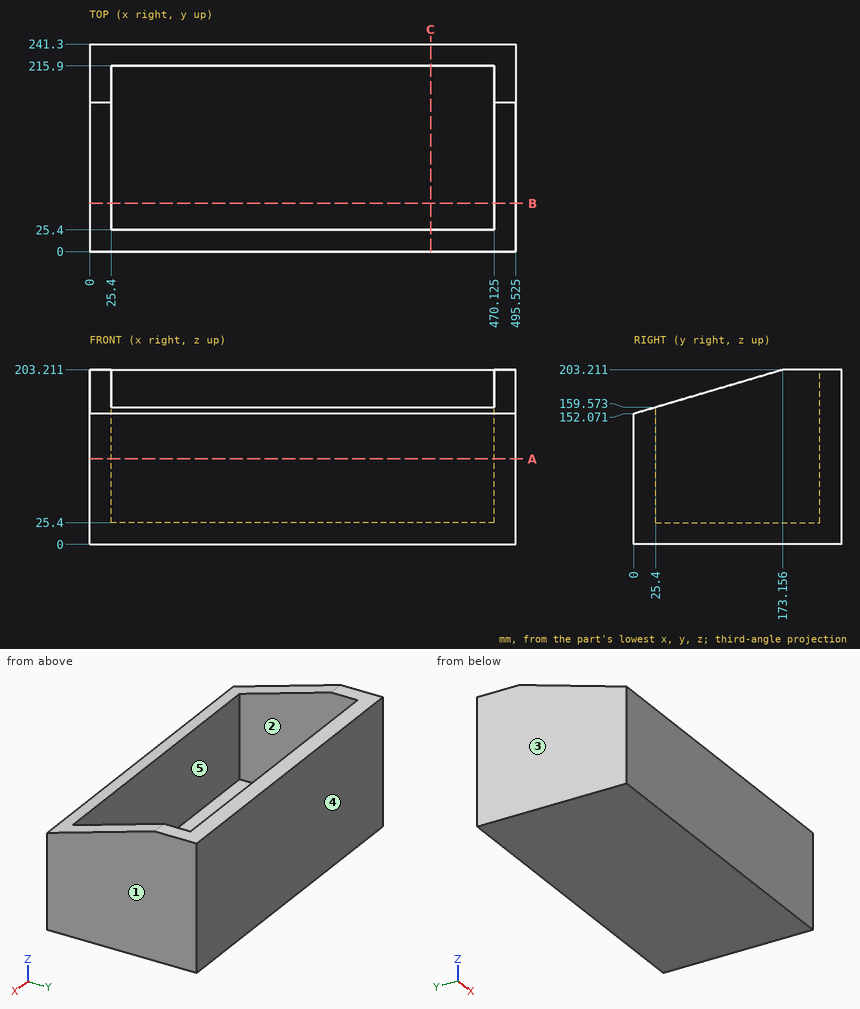
Design review of the part shown in the three views and the two pictorial views. Dimensions are in mm from the part's minimum x, y and z. A direction names the side the tool comes from. Give positions to 0.01 mm unless a question says otherwise; leave off trailing zeros. Loops run counter-clockwise (first coordinate to the right, second up) from the corner with the lowest first, then second, coordinate; pieces in that order, holes last. Notation, with made-up numbers: (53.5, -9.75) -> (107.5, -9.75) arc R19 ccw to (107.5, 8.25) -> close; hole circle Ø7 at (-2, 8.25). An arc over 180 degrees is marked (long way). Write each question's results on one line, items separated by ' | '.
1) Take a section at A-A, the plane z = 99.5. Give the boundary of the cut face in (x, y) (1 decimal), plus the area to 4 significant figures.
Conclusion:
outline: (0, 0) -> (495.5, 0) -> (495.5, 241.3) -> (0, 241.3) -> close; hole (25.4, 25.4) -> (470.1, 25.4) -> (470.1, 215.9) -> (25.4, 215.9) -> close | area: 34,850 mm^2
2) Take a section at B-B, the plane y = 56. Give the boundary of the cut face in (x, z) (1 decimal), plus the area to 3 significant figures.
Conclusion:
outline: (0, 0) -> (495.5, 0) -> (495.5, 168.6) -> (470.1, 168.6) -> (470.1, 25.4) -> (25.4, 25.4) -> (25.4, 168.6) -> (0, 168.6) -> close | area: 19,900 mm^2
3) Take a section at C-C, the plane x = 396.5. Give the boundary of the cut face in (y, z).
Conclusion:
outline: (0, 0) -> (241.3, 0) -> (241.3, 203.21) -> (215.9, 203.21) -> (215.9, 25.4) -> (25.4, 25.4) -> (25.4, 159.57) -> (0, 152.07) -> close
4) Insertion check: pin 1 Ø1.5 at (x, y) = (266.5, 96.5) entering from +Z. The pin has a flat end and moves straight along its axis. Give the tip position at first contact, or say it passes through.
Conclusion:
pin 1: stops at z = 25.4
5) For line 1 along X through (y, z) = (159, 112.5) (1 decimal); line 2 along Y through (x, z) = (83.5, 143.5); line 3 along Z through (x, y) = (44, 55.5), list the stretches that pass through material, from the lowest coordinate up. Write a range as from..to.
Conclusion:
line 1: x = 0..25.4, 470.1..495.5 | line 2: y = 0..25.4, 215.9..241.3 | line 3: z = 0..25.4
6) Draft analysis for pull direction X (two halves, no side actions). For the marked faces 1, 2 and 3, state which applies: pulls with the +X half, pulls with the -X half, needs draft (parallel to the pull), parting line crosses it, or undercut.
Conclusion:
face 1: pulls with the +X half | face 2: undercut | face 3: pulls with the -X half
7) Tool access review of the marked faces 4 and 5: name each direction out of +Z, -Z, +X, -X, +Y, -Y from which nothing blocks a thin tool from reaching the whole face with its end or side.
Conclusion:
face 4: +Z, -Z, +X, -X, +Y | face 5: +Z
